from build123d import *

# Parameters (mm, degrees)
BOSS_EXTRUDE1_DEPTH = 6.35
SKETCH20_R          = 35
BOSS_EXTRUDE5_DEPTH = 19.05
CUT_EXTRUDE14_DEPTH = 123.39448517
CHAMFER1_SIZE       = 19.05
SKETCH22_R          = 3.175
CUT_EXTRUDE15_DEPTH = 129.555411344
SKETCH24_R          = 5
CUT_EXTRUDE16_DEPTH = 134.419011414
SKETCH25_R          = 2.38125
CUT_EXTRUDE17_DEPTH = 10
CUT_EXTRUDE18_DEPTH = 10
CHAMFER3_SIZE       = 2.5
FILLET1_R           = 1.5875


with BuildPart() as part:
    # Sketch1 → Boss-Extrude1 (new body)
    with BuildSketch(Plane(origin=(0, 0, 0), x_dir=(0, 0, -1), z_dir=(1, 0, 0))):
        with BuildLine():
            Line((-34.853407294, -3.2), (-26.886914198, -89.968571429))
            ThreePointArc((-26.886914198, -89.968571429), (0, -114.5), (26.886914198, -89.968571429))
            Line((26.886914198, -89.968571429), (34.853407294, -3.2))
            ThreePointArc((34.853407294, -3.2), (0, 35), (-34.853407294, -3.2))
        make_face()
        Polygon((4.353205728, 11.960334439), (-11.960334439, 4.353205728), (-4.353205728, -11.960334439), (11.960334439, -4.353205728), align=None, mode=Mode.SUBTRACT)
    extrude(amount=BOSS_EXTRUDE1_DEPTH)

    # Sketch20 → Boss-Extrude5 (add)
    with BuildSketch(Plane(origin=(6.35, 0, 0), x_dir=(0, 0, -1), z_dir=(1, 0, 0))):
        with Locations(Location((0, 0, 0), (0, 0, 185.245797084))):
            Circle(SKETCH20_R)
    extrude(amount=BOSS_EXTRUDE5_DEPTH)

    # Sketch21 → Cut-Extrude14 (cut, through all)
    with BuildSketch(Plane.ZY):
        Polygon((-19.067760927, 15.897892729), (-24.435012851, 4.387783834), (-10.840396045, -1.951490092), (-5.473144121, 9.558618803), align=None)
        Polygon((-11.960334439, -4.353205728), (-4.353205728, 11.960334439), (11.960334439, 4.353205728), (4.353205728, -11.960334439), align=None)
        Polygon((10.840396045, 1.951490092), (5.473144121, -9.558618803), (19.067760927, -15.897892729), (24.435012851, -4.387783834), align=None)
    extrude(amount=-CUT_EXTRUDE14_DEPTH, mode=Mode.SUBTRACT)

    # Chamfer1
    # the kernel refuses this chamfer: 19.05 mm, written as the material it takes off along each edge
    with BuildSketch(Plane(origin=(25.4, 0, 0), x_dir=(0, -0.09142857142327497, 0.9958116369713196), z_dir=(0, 0.9958116369713196, 0.09142857142327497))) as chamfer1_piece_1:
        Polygon((35 - CHAMFER1_SIZE, 0), (35, -CHAMFER1_SIZE), (35, 0), align=None)
    revolve(axis=Axis((25.4, 0, 0), (1, 0, 0)), mode=Mode.SUBTRACT)

    # Sketch22 → Cut-Extrude15 (cut, through all)
    with BuildSketch(Plane(origin=(0, 5.755054448, 2.683625962), x_dir=(-1, 0, 0), z_dir=(0, -0.9063077870366495, -0.4226182617407006))):
        with Locations(Location((-13.4, -16.5, 0), (0, 0, 90))):
            Circle(SKETCH22_R)
    cut_extrude15 = extrude(amount=-CUT_EXTRUDE15_DEPTH, mode=Mode.SUBTRACT)

    # Sketch24 → Cut-Extrude16 (cut, through all)
    with BuildSketch(Plane(origin=(0, 10.286593383, 4.796717271), x_dir=(-1, 0, 0), z_dir=(0, -0.9063077870366495, -0.4226182617407006))):
        with Locations(Location((-13.4, -16.5, 0), (0, 0, 90))):
            Circle(SKETCH24_R)
    cut_extrude16 = extrude(amount=-CUT_EXTRUDE16_DEPTH, mode=Mode.SUBTRACT)

    # Sketch25 → Cut-Extrude17 (cut)
    with BuildSketch(Plane(origin=(0, -5.755054448, -2.683625962), x_dir=(1, 0, 0), z_dir=(0, 0.9063077870366495, 0.4226182617407006))):
        with Locations(Location((13.4, -16.5, 0), (0, 0, 270))):
            Circle(SKETCH25_R)
    cut_extrude17 = extrude(amount=-CUT_EXTRUDE17_DEPTH, mode=Mode.SUBTRACT)

    # Mirror1: Cut-Extrude15, Cut-Extrude16, Cut-Extrude17 across plane
    add(cut_extrude15.mirror(Plane(origin=(0, 0, 0), x_dir=(1, 0, 0), z_dir=(0, 0.422618261740701, -0.9063077870366492))), mode=Mode.SUBTRACT)
    add(cut_extrude16.mirror(Plane(origin=(0, 0, 0), x_dir=(1, 0, 0), z_dir=(0, 0.422618261740701, -0.9063077870366492))), mode=Mode.SUBTRACT)
    add(cut_extrude17.mirror(Plane(origin=(0, 0, 0), x_dir=(1, 0, 0), z_dir=(0, 0.422618261740701, -0.9063077870366492))), mode=Mode.SUBTRACT)

    # Sketch19 → Cut-Extrude18 (cut)
    with BuildSketch(Plane(origin=(6.35, 0, 0), x_dir=(0, 0, -1), z_dir=(1, 0, 0))):
        with BuildLine():
            Line((13.556349186, -66.943650814), (13.556349186, -71.943650814))
            ThreePointArc((13.556349186, -71.943650814), (15.556349186, -73.943650814), (17.556349186, -71.943650814))
            Line((17.556349186, -71.943650814), (17.556349186, -66.943650814))
            ThreePointArc((17.556349186, -66.943650814), (15.556349186, -64.943650814), (13.556349186, -66.943650814))
        make_face()
        with BuildLine():
            Line((-10, -82.5), (-10, -87.5))
            ThreePointArc((-10, -87.5), (0, -97.5), (10, -87.5))
            Line((10, -87.5), (10, -82.5))
            ThreePointArc((10, -82.5), (0, -72.5), (-10, -82.5))
        make_face()
        with BuildLine():
            Line((17.556349186, -103.056349186), (17.556349186, -98.056349186))
            ThreePointArc((17.556349186, -98.056349186), (15.556349186, -96.056349186), (13.556349186, -98.056349186))
            Line((13.556349186, -98.056349186), (13.556349186, -103.056349186))
            ThreePointArc((13.556349186, -103.056349186), (15.556349186, -105.056349186), (17.556349186, -103.056349186))
        make_face()
        with BuildLine():
            Line((-17.556349186, -66.943650814), (-17.556349186, -71.943650814))
            ThreePointArc((-17.556349186, -71.943650814), (-15.556349186, -73.943650814), (-13.556349186, -71.943650814))
            Line((-13.556349186, -71.943650814), (-13.556349186, -66.943650814))
            ThreePointArc((-13.556349186, -66.943650814), (-15.556349186, -64.943650814), (-17.556349186, -66.943650814))
        make_face()
        with BuildLine():
            Line((-13.556349186, -103.056349186), (-13.556349186, -98.056349186))
            ThreePointArc((-13.556349186, -98.056349186), (-15.556349186, -96.056349186), (-17.556349186, -98.056349186))
            Line((-17.556349186, -98.056349186), (-17.556349186, -103.056349186))
            ThreePointArc((-17.556349186, -103.056349186), (-15.556349186, -105.056349186), (-13.556349186, -103.056349186))
        make_face()
    extrude(amount=-CUT_EXTRUDE18_DEPTH, mode=Mode.SUBTRACT)


with BuildPart() as body_2:
    # Mirror2: mirrored copy
    add(part.part.mirror(Plane(origin=(0, 0, 0), x_dir=(0, 0, 1), z_dir=(1, 0, 0))))

    # Chamfer3
    chamfer3_edges = [body_2.edges().sort_by_distance(p)[0] for p in [
        (0, -69.443650814, 13.556349186),
        (0, -64.943650814, 15.556349186),
        (0, -69.443650814, 17.556349186),
        (0, -73.943650814, 15.556349186),
        (0, -69.443650814, -17.556349186),
        (0, -64.943650814, -15.556349186),
        (0, -69.443650814, -13.556349186),
        (0, -73.943650814, -15.556349186),
    ]]
    chamfer(chamfer3_edges, length=CHAMFER3_SIZE)

    # Fillet1
    fillet1_edges = [body_2.edges().sort_by_distance(p)[0] for p in [
        (-8.262078305, 4.387783834, -24.435012851),
        (-8.262078305, 15.897892729, -19.067760927),
        (-8.262078305, -4.387783834, 24.435012851),
        (-8.262078305, -15.897892729, 19.067760927),
        (-12.7, 11.960334439, -4.353205728),
        (-12.7, 4.353205728, 11.960334439),
        (-12.7, -11.960334439, 4.353205728),
        (-12.7, -4.353205728, -11.960334439),
    ]]
    fillet(fillet1_edges, radius=FILLET1_R)


solid = body_2.part
Source: CAD feature listing. Evaluate the final solid. Frame: model axes, mm. A direction names the side the tool comes from. Coordinates: 2 decimals unless noted, no trailing zeros. Write each question's results on one line, items separated by ' | '. Start each with the question number.
Item 1: Set-up query: faces 5 (the face through (-10.14, 3.75, 18.81)), 6 (the face through (-3, -101, 17.556)), 7 (the face through (-1.788, -64.232, -15.616)). Return all of +Z, -Z, +X, -X, +Y, -Y with unobstructed straight access to the full face (end or side cutting, diameter ignored); none if empty.
Item 2: First-contact query: pin 1 Ø3 at (x, z) = (-7, 21) entering from -Y; pin 2 Ø5 at (x, y) = (-10, 13) entering from +Z; pin 3 Ø1.2 at (x, y) = (-4, -70.5) entering from +Z. Flat tips, straight axial feed; report the tip coordinate or a pass-through.
Item 3: Cut plane A-A (z = 8). Count the separate pieces of the cut face and the enclosed holes in it, and give its area (3 significant figures).
Item 4: Draft query along Z for faces 1 (the face through (-24.21, -10.38, -13.64)), 2 (the face through (-15.76, -17.07, 9.91)), 3 (the face through (-3.2, -72.5, -0.2)), 4 (the face through (-6.35, -70, 0)). Return one class per face: pulls with the +Z half, pulls with the -Z half, needs draft (parallel to the pull), parting line crosses it, or undercut.
Item 5: Line query: probe 1 along X at (y, z) = (-38.5, 10.5); probe 2 along Y at (x, z) = (-6.5, 11); probe 3 along Y at (x, z) = (-17, -13). Output: solid intervals per line, ascending.
Checked values:
1) face 5: none | face 6: +X, -X | face 7: +X
2) pin 1: stops at y = -106.02 | pin 2: stops at z = 31.43 | pin 3: stops at z = 28.73
3) separate pieces: 3 | enclosed holes: 1 | area: 1,300 mm2
4) face 1: parting line crosses it | face 2: undercut | face 3: undercut | face 4: needs draft
5) probe 1: x = -6.35 to 0 | probe 2: y = -33.07 to -12.14, 1.88 to 2.29, 4.68 to 33.07 | probe 3: y = -20.59 to -0.94, 13.07 to 18.59, 19.37 to 20.59
